```python
from build123d import *

# Parameters (mm, degrees)
SKETCH1_W           = 55.7
SKETCH1_H           = 31.7
BOSS_EXTRUDE1_DEPTH = 13.7
SKETCH2_W           = 14.5
SKETCH2_H           = 27
CUT_EXTRUDE1_DEPTH  = 13.7
SKETCH3_W           = 51.7
SKETCH3_H           = 27.7
CUT_EXTRUDE2_DEPTH  = 13


with BuildPart() as part:
    # Sketch1 → Boss-Extrude1 (new body)
    with BuildSketch(Plane(origin=(0, 0, 0), x_dir=(1, 0, 0), z_dir=(0, 1, 0))):
        with Locations((27.85, 15.85)):
            Rectangle(SKETCH1_W, SKETCH1_H)
    extrude(amount=BOSS_EXTRUDE1_DEPTH)

    # Sketch2 → Cut-Extrude1 (cut)
    with BuildSketch(Plane(origin=(0, 13.7, 0), x_dir=(1, 0, 0), z_dir=(0, 1, 0))):
        with Locations((41.95, 15.85)):
            Rectangle(SKETCH2_W, SKETCH2_H)
    extrude(amount=-CUT_EXTRUDE1_DEPTH, mode=Mode.SUBTRACT)

    # Sketch3 → Cut-Extrude2 (cut)
    with BuildSketch(Plane.XZ):
        with Locations((27.85, -15.85)):
            Rectangle(SKETCH3_W, SKETCH3_H)
    extrude(amount=-CUT_EXTRUDE2_DEPTH, mode=Mode.SUBTRACT)


solid = part.part
```
Verification items for the finished model (mm, model axes). A direction names the side the tool comes from. Give positions to 0.01 mm unless a question says otherwise; leave off trailing zeros. Order: outer loops, then holes, each group sorted by start corner. A loop starts at its lowest first (then second) coordinate and runs counter-clockwise, first axis right, second up. Notation, with made-up numbers: M 38.5,25.5 L 82.5,25.5 A24 cw 82.5,48.5 Z; hole C 17,57.25 d7. An arc over 180 degrees is marked long. Answer in a Markdown table with one row per item. Add a question column.
Item 1: Section check A-A, the plane x = 39. Enter the section's corners in (y, z).
Item 2: Section check D-D, the plane x = 16. Enter the section's corners in (y, z), and give its area (3 significant figures).
Item 3: Section check C-C, the plane z = -6.5. Enter the section's corners in (x, y).
Item 4: Scan lines: probe 1 along X at (y, z) = (10.5, -20.5); probe 2 along Z at (x, y) = (31, 2.5); probe 3 along Y at (x, z) = (10, -18). Record each from-to range of solid material in increasing order. Write a range as from..to.
Item 5: Gauge pin test, flat end, axial feed: pin 1 (12 mm diameter, centred on x = 46.5, z = -20.5, fed in from -Y). Record the tip position at first contact, or that the pin passes through.
Item 6: Mould release check, pull along Z, two halves, no side actions. Record for faces 3 (the flat face through (53.7, 6, -16)), 4 (the flat face through (55.7, 7, -16)), 5 (the flat face through (27, 7, -31.7)): released by +Z, released by -Z, zero draft, split by the parting line, or undercut.
Item 7: Section check B-B, the plane y = 10. Enter the section's corners in (x, z).
Item 8: Tool access check on faces 1 (the flat face through (21, 13.7, -16)), 2 (the flat face through (27, 6, -29.7)). Record the directions out of +Z, -Z, +X, -X, +Y, -Y that give a thin tool (end or side, any length) a straight path to the whole face; none if there is none.
Filled sheet:
| question | item | result |
|---|---|---|
| 1 | outline | M 0,-31.7 L 13.7,-31.7 L 13.7,-29.35 L 13,-29.35 L 13,-29.7 L 0,-29.7 Z; M 0,-2 L 13,-2 L 13,-2.35 L 13.7,-2.35 L 13.7,0 L 0,0 Z |
| 2 | outline | M 0,-31.7 L 13.7,-31.7 L 13.7,0 L 0,0 L 0,-2 L 13,-2 L 13,-29.7 L 0,-29.7 Z |
| 2 | area | 74.2 mm^2 |
| 3 | outline | M 0,0 L 2,0 L 2,13 L 34.7,13 L 34.7,13.7 L 0,13.7 Z; M 49.2,13 L 53.7,13 L 53.7,0 L 55.7,0 L 55.7,13.7 L 49.2,13.7 Z |
| 4 | probe 1 | x = 0..2, 53.7..55.7 |
| 4 | probe 2 | z = -31.7..-29.7, -2..0 |
| 4 | probe 3 | y = 13..13.7 |
| 5 | pin 1 | stops at y = 13 |
| 6 | face 3 | undercut |
| 6 | face 4 | zero draft |
| 6 | face 5 | released by -Z |
| 7 | outline | M 0,-31.7 L 55.7,-31.7 L 55.7,0 L 0,0 Z; hole M 2,-29.7 L 53.7,-29.7 L 53.7,-2 L 2,-2 Z |
| 8 | face 1 | +Z, -Z, +X, -X, +Y |
| 8 | face 2 | -Y |
